```python
from build123d import *

# Parameters (mm, degrees)
EXTRUDE_1_DEPTH          = 5
CUT_EXTRUDE_3_DEPTH      = 31.822070015
CUT_EXTRUDE_3_DEPTH_BACK = 31.822070015
SKETCH_5_R               = 1.05


with BuildPart() as part:
    # ｽｹｯﾁ1 → ﾎﾞｽ - 押し出し1 (new body)
    with BuildSketch(Plane.XY):
        with BuildLine():
            ThreePointArc((-25, 5), (-30, 0), (-25, -5))
            Line((-25, -5), (-25, 5))
        make_face()
        with BuildLine():
            Line((-25, 5), (-25, -5))
            ThreePointArc((-25, -5), (-21.464466094, -3.535533906), (-20, 0))
            ThreePointArc((-20, 0), (-21.464466094, 3.535533906), (-25, 5))
        make_face()
        with BuildLine():
            ThreePointArc((-20, 0), (-21.464466094, -3.535533906), (-25, -5))
            Line((-25, -5), (25, -5))
            ThreePointArc((25, -5), (20, 0), (25, 5))
            Line((25, 5), (-25, 5))
            ThreePointArc((-25, 5), (-21.464466094, 3.535533906), (-20, 0))
        make_face()
        with BuildLine():
            ThreePointArc((25, 5), (20, 0), (25, -5))
            Line((25, -5), (25, 5))
        make_face()
        with BuildLine():
            Line((25, 5), (25, -5))
            ThreePointArc((25, -5), (28.535533906, -3.535533906), (30, 0))
            ThreePointArc((30, 0), (28.535533906, 3.535533906), (25, 5))
        make_face()
    extrude(amount=EXTRUDE_1_DEPTH)

    # ｽｹｯﾁ5 → ｶｯﾄ - 押し出し3 (cut, two sides: drawn at the far end of the back side and taken through both)
    with BuildSketch(Plane.XY.offset(-CUT_EXTRUDE_3_DEPTH_BACK)):
        with Locations((25, 0)):
            Circle(SKETCH_5_R)
        with Locations((-25, 0)):
            Circle(SKETCH_5_R)
    extrude(amount=CUT_EXTRUDE_3_DEPTH + CUT_EXTRUDE_3_DEPTH_BACK, mode=Mode.SUBTRACT)


solid = part.part
```
Read the model definition and answer for the solid it produces. Units are mm, in the model's axes. Coordinates: 2 decimals unless noted, no trailing zeros. Loops run counter-clockwise (first coordinate to the right, second up) from the corner with the lowest first, then second, coordinate; pieces in that order, holes last.
(1) Consider line 1 along X through (y, z) = (0, 3.6); line 2 along Y through (x, z) = (25, 2.75); line 3 along X through (y, z) = (3, 3.8). Determine where each line is inside the solid, lowest interval first.
Solution:
line 1: x = -30 to -26.05, -23.95 to 23.95, 26.05 to 30
line 2: y = -5 to -1.05, 1.05 to 5
line 3: x = -29 to 29
(2) The part is cut by section C-C (y = -2.25). Determine the outline of the cut face in (x, z), and give its area (3 significant figures).
Solution:
outline: (-29.47, 0) - (29.47, 0) - (29.47, 5) - (-29.47, 5) - close
area: 295 mm2
(3) The part is cut by section A-A (z = 2.8). Determine the outline of the cut face in (x, y).
Solution:
outline: (-25, -5) - (25, -5) arc R5 ccw to (25, 5) - (-25, 5) arc R5 ccw to start; hole circle Ø2.1 at (-25, 0); hole circle Ø2.1 at (25, 0)
(4) The mould has two halves that part along Y. Classify faces 1 (the face through (0, 5, 2)), 2 (the face through (0, -5, 2)), 3 (the face through (25.97, -0.4, 2.46)): released by +Y, released by -Y, zero draft, split by the parting line, or undercut.
Solution:
face 1: released by +Y
face 2: released by -Y
face 3: undercut
(5) The part is cut by section B-B (y = 3). Determine the outline of the cut face in (x, z), and give its area (3 significant figures).
Solution:
outline: (-29, 0) - (29, 0) - (29, 5) - (-29, 5) - close
area: 290 mm2
